Verification items for the finished model (mm, model axes). A direction names the side the tool comes from. Coordinates: 2 decimals unless noted, no trailing zeros. Write item = value, one per line. Start each with the question number.
(1) Gauge pin test, flat ends, axial feed: pin 1 Ø3 at (x, y) = (-1, 2.5) entering from -Z; pin 2 Ø1 at (y, z) = (0, 1) entering from -X; pin 3 Ø1 at (y, z) = (-1.5, -1) entering from +X; pin 4 Ø0.9 at (y, z) = (0.5, 0.5) entering from -X. Record the tip position at first contact, or that the pin passes through.
(2) Mould release check, pull along Y, two halves, no side actions. Record for faces 4 (the face through (0.87, -1.47, 1.46)), 5 (the face through (-2.2, 1.58, -1.42)), 6 (the face through (2, 0, -1.588)): released by +Y, released by -Y, zero draft, split by the parting line, or undercut.
(3) Material ranges on probe 1 along Z at (x, y) = (-1.75, -2); probe 2 along Z at (x, y) = (-2.5, 0.25); probe 3 along X at (y, z) = (-0.5, -1), recorded low to high. Write a range as [from, to].
(4) Set-up check for faces 1 (the face through (0.8, 1.37, 0.02)), 2 (the face through (-2, -1, 1.588)), 3 (the face through (-0.87, 1.47, 1.46)): record each of +Z, -Z, +X, -X, +Y, -Y from which the full face is reachable in a straight line by a thin tool's end or side.
```python
from build123d import *

# Parameters (mm, degrees)
CUT_SWEEP2_PITCH    = 1.27
CUT_EXTRUDE10_DEPTH = 6.499261487


with BuildPart() as part:
    # Sketch22 → Revolve1 (revolve)
    with BuildSketch(Plane(origin=(0, 0, 0), x_dir=(0, 0, -1), z_dir=(1, 0, 0)), mode=Mode.PRIVATE) as revolve1_sk:
        Polygon((-1.5875, 0), (-1.5875, 2.54), (-1.142868213, 3.175), (0.9525, 3.175), (1.5875, 2.54), (1.5875, 0), (0, 0), align=None)
    revolve(revolve1_sk.sketch.rotate(Axis((0, 0, 0), (0, 0, -1)), 180), axis=Axis((0, 0, 0), (0, 0, -1)))

    # Cut-Sweep2: the profile of Sketch28 profile screwed along a right-hand helix of 3.5 turns, 8 arcs to a turn; built about Z, then put on its axis
    cut_sweep2_z = Axis((0, 0, 0), (0, 0, 1))
    cut_sweep2_corners = [(3.1753, 0, 0.000173205), (3.1753, 0, -1.111423205), (2.350110803, 0, -0.635), (2.350110803, 0, -0.47625)]
    with BuildLine(mode=Mode.PRIVATE) as cut_sweep2_profile:
        Line(cut_sweep2_corners[0], cut_sweep2_corners[1])
        Line(cut_sweep2_corners[1], cut_sweep2_corners[2])
        Line(cut_sweep2_corners[2], cut_sweep2_corners[3])
        Line(cut_sweep2_corners[3], cut_sweep2_corners[0])
    cut_sweep2_cap = Face(cut_sweep2_profile.wire())
    cut_sweep2_turn_angles = [0, 22.5, 45, 67.5, 90, 112.5, 135, 157.5, 180, 202.5, 225, 247.5, 270, 292.5, 315, 337.5, 360]
    cut_sweep2_turn_weights = [1, 0.9238795325112867, 1, 0.9238795325112867, 1, 0.9238795325112867, 1, 0.9238795325112867, 1, 0.9238795325112867, 1, 0.9238795325112867, 1, 0.9238795325112867, 1, 0.9238795325112867, 1]
    cut_sweep2_turn_rails = [Edge.make_bspline([Vector(p[0], p[1], 0).rotate(cut_sweep2_z, cut_sweep2_turn_angles[k]) / cut_sweep2_turn_weights[k] + Vector(0, 0, p[2] + CUT_SWEEP2_PITCH * cut_sweep2_turn_angles[k] / 360) for k in range(17)], [0, 0, 0, 1, 1, 2, 2, 3, 3, 4, 4, 5, 5, 6, 6, 7, 7, 8, 8, 8], 2, cut_sweep2_turn_weights) for p in cut_sweep2_corners]
    cut_sweep2_turn_sides = [Face.make_surface_from_curves(cut_sweep2_turn_rails[p[0]], cut_sweep2_turn_rails[p[1]]) for p in [(0, 1), (1, 2), (2, 3), (3, 0)]]
    cut_sweep2_last_angles = [1080, 1102.5, 1125, 1147.5, 1170, 1192.5, 1215, 1237.5, 1260]
    cut_sweep2_last_weights = [1, 0.9238795325112867, 1, 0.9238795325112867, 1, 0.9238795325112867, 1, 0.9238795325112769, 1]
    cut_sweep2_last_rails = [Edge.make_bspline([Vector(p[0], p[1], 0).rotate(cut_sweep2_z, cut_sweep2_last_angles[k]) / cut_sweep2_last_weights[k] + Vector(0, 0, p[2] + CUT_SWEEP2_PITCH * cut_sweep2_last_angles[k] / 360) for k in range(9)], [0, 0, 0, 1, 1, 2, 2, 3, 3, 4, 4, 4], 2, cut_sweep2_last_weights) for p in cut_sweep2_corners]
    cut_sweep2_last_sides = [Face.make_surface_from_curves(cut_sweep2_last_rails[p[0]], cut_sweep2_last_rails[p[1]]) for p in [(0, 1), (1, 2), (2, 3), (3, 0)]]
    cut_sweep2 = Plane(origin=(0, 0, -1.5875), x_dir=(0, 1, 0), z_dir=(0, 0, 1)) * Solid(Shell([*[p.moved(Location((0, 0, CUT_SWEEP2_PITCH * i))) for i in range(3) for p in cut_sweep2_turn_sides], *cut_sweep2_last_sides, cut_sweep2_cap, cut_sweep2_cap.rotate(cut_sweep2_z, 1260).moved(Location((0, 0, CUT_SWEEP2_PITCH * 1260 / 360)))]))
    add(cut_sweep2, mode=Mode.SUBTRACT)

    # Sketch23 → Cut-Extrude10 (cut, through all)
    with BuildSketch(Plane.XY.offset(1.5875)):
        Polygon((0, 1.833087105), (-1.5875, 0.916543552), (-1.5875, -0.916543552), (0, -1.833087105), (1.5875, -0.916543552), (1.5875, 0.916543552), align=None)
    extrude(amount=-CUT_EXTRUDE10_DEPTH, mode=Mode.SUBTRACT)

    # Cut-Extrude11 cone 1 section (through the dimple's axis) → Cut-Extrude11 (revolve, cut)
    with BuildSketch(Plane(origin=(0, 0, 1.5875), x_dir=(0, -1, 0), z_dir=(1, 0, 0))):
        Polygon((0, 0), (1.833087105, 0), (0, 1.833087105), align=None)
    revolve(axis=Axis((0, 0, 1.5875), (0, 0, -1)), mode=Mode.SUBTRACT)


solid = part.part
```
Response:
q1.pin_1 = -1.59
q1.pin_2 = -3.08
q1.pin_3 = 2.98
q1.pin_4 = -3.17
q2.face_4 = undercut
q2.face_5 = split by the parting line
q2.face_6 = zero draft
q3.probe_1 = [-1.4, -0.64], [-0.13, 0.63], [1.14, 1.51]
q3.probe_2 = [-1.59, -0.75], [-0.4, 0.52], [0.87, 1.59]
q3.probe_3 = [-3, -1.59], [1.59, 2.56]
q4.face_1 = +Z, -Z
q4.face_2 = +Z, +X, -X, +Y, -Y
q4.face_3 = +Z
